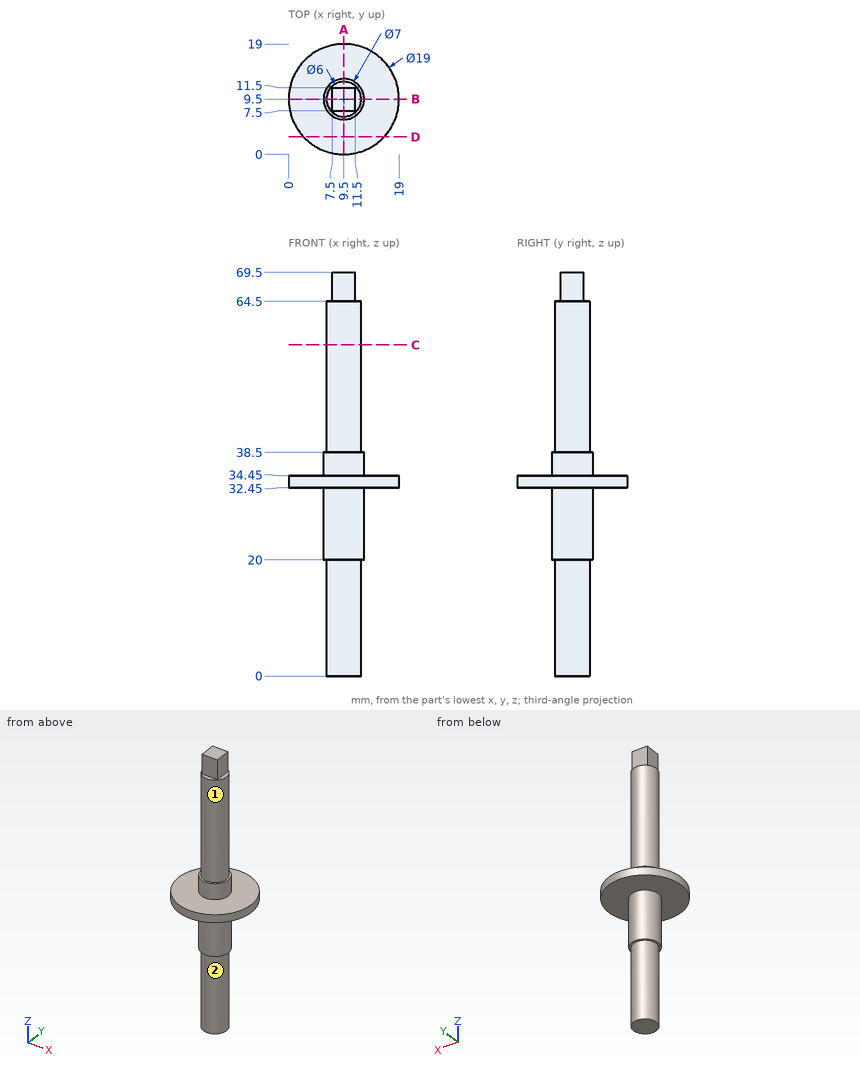
Source: three-view drawing plus pictorial views. Frame: mm from the lowest corner of the part. A direction names the side the tool comes from. Round coordinates to 2 decimals unless told otherwise and drop trailing zeros. Loops run counter-clockwise (first coordinate to the right, second up) from the corner with the lowest first, then second, coordinate; pieces in that order, holes last. Notation, with made-up numbers: M 58.5,83.25 L 103.5,83.25 A26 cw 103.5,113.25 Z; hole C -33,54.5 d4. An arc over 180 degrees is marked long. Answer as CSV lines item,"result".
Q1. Contact query for flat-ended pins moving along their axis: pin 1 (8 mm diameter, centred on x = 14, y = 2.5, fed in from -Z); pin 2 (10 mm diameter, centred on y = 5.5, z = 43.5, fed in from +X); pin 3 (6 mm diameter, centred on x = 8, z = 25.5, fed in from +Y); pin 4 (1 mm diameter, centred on x = 5, z = 49.5, fed in from +Y). Output: stop coordinate, or through.
Verdict:
pin 1,"stops at z = 32.45"
pin 2,"stops at x = 12.5"
pin 3,"stops at y = 13"
pin 4,"passes through"
Q2. Cut plane D-D (y = 3). Return the cut outline in (x, z).
Verdict:
outline,"M 2.57,32.45 L 16.43,32.45 L 16.43,34.45 L 2.57,34.45 Z"
Q3. Cut plane C-C (z = 57). Return the cut outline in (x, y).
Verdict:
outline,"C 9.5,9.5 d6"
Q4. Line query: line 1 along Z through (x, y) = (6.25, 2.25); line 2 along Z through (x, y) = (6.5, 8.75); line 3 along X through (y, z) = (9.75, 47.5). Output: solid intervals per line, ascending.
Verdict:
line 1,"z = 32.45 to 34.45"
line 2,"z = 20 to 38.5"
line 3,"x = 6.51 to 12.49"
Q5. Reachability of the marked faces 1 and 2 from +Z, -Z, +X, -X, +Y, -Y: full face, straight path, thin tool, end or side. Return the list, or none.
Verdict:
face 1,"+Z"
face 2,"-Z"
Q6. Cut plane A-A (x = 9.5). Return the cut outline in (y, z), plus the area to 4 significant figures.
Verdict:
outline,"M 0,32.45 L 6,32.45 L 6,20 L 6.5,20 L 6.5,0 L 12.5,0 L 12.5,20 L 13,20 L 13,32.45 L 19,32.45 L 19,34.45 L 13,34.45 L 13,38.5 L 12.5,38.5 L 12.5,64.5 L 11.5,64.5 L 11.5,69.5 L 7.5,69.5 L 7.5,64.5 L 6.5,64.5 L 6.5,38.5 L 6,38.5 L 6,34.45 L 0,34.45 Z"
area,"449.5 mm^2"
